Read the model definition and answer for the solid it produces. Units are mm, in the model's axes. A direction names the side the tool comes from. Round coordinates to 2 decimals unless told otherwise and drop trailing zeros. Write each loop counter-clockwise with the first axis right and the second up, starting at its lowest first coordinate (ties: lowest second). Pieces come first, ordered by that corner, then holes. Notation, with made-up numbers: (52.5, 2.25) -> (63.5, 2.25) arc R25 ccw to (63.5, 27.25) -> close; hole circle Ø3 at (85, 34). An arc over 180 degrees is marked (long way). Return JSON: item names as keys, results as strings.
Autodesk Inventor part; units mm, degrees
ref_plane "YZ Plane" through (0, 0, 0) normal (1, 0, 0) x (0, 1, 0)
ref_plane "XZ Plane" through (0, 0, 0) normal (0, 1, 0) x (-1, 0, 0)
ref_plane "XY Plane" through (0, 0, 0) normal (0, 0, 1) x (1, 0, 0)
sketch "스케치1" plane through (0, 0, 0) normal (0, 1, 0) x (-1, 0, 0)
  line L0 (17.6385, -30.5508) -> (-17.6385, -30.5508)
  line L1 (-17.6385, -30.5508) -> (-35.277, 0)
  line L2 (-35.277, 0) -> (-17.6385, 30.5508)
  line L3 (-17.6385, 30.5508) -> (17.6385, 30.5508)
  line L4 (17.6385, 30.5508) -> (35.277, 0)
  line L5 (35.277, 0) -> (17.6385, -30.5508)
  line L6 (19.486, -33.7508) -> (-19.486, -33.7508)
  line L7 (-19.486, -33.7508) -> (-38.972, 0)
  line L8 (-38.972, 0) -> (-19.486, 33.7508)
  line L9 (-19.486, 33.7508) -> (19.486, 33.7508)
  line L10 (19.486, 33.7508) -> (38.972, 0)
  line L11 (38.972, 0) -> (19.486, -33.7508)
  point P0 (0, 0)
  point P1 (0, 0)
  point P2 (0, 0)
  dimension "d0" = 70.554
  dimension "d1" = 3.2
extrude "돌출1" add sketch "스케치1" along normal blind 3.7 contours L0 L1 L2 L3 L4 L5 | L6 L7 L8 L9 L10 L11
sketch "스케치2" plane through (0, 3.7, 0) normal (0, 1, 0) x (1, 0, 0)
  line L0 (-18.5623, 32.1508) -> (18.5623, 32.1508)
  line L1 (18.5623, 32.1508) -> (37.1245, 0)
  line L2 (37.1245, 0) -> (18.5623, -32.1508)
  line L3 (18.5623, -32.1508) -> (-18.5623, -32.1508)
  line L4 (-18.5623, -32.1508) -> (-37.1245, 0)
  line L5 (-37.1245, 0) -> (-18.5623, 32.1508)
  line L6 (-19.486, 33.7508) -> (-38.972, 0)
  point P0 (0, 0)
  point P1 (0, 0)
  dimension "d4" = 1.6
extrude "돌출2" cut sketch "스케치2" against normal blind 1.2
sketch "스케치3" plane through (0, 2.5, 0) normal (0, 1, 0) x (1, 0, 0)
  line L0 (17.4076, -30.1508) -> (-17.4076, -30.1508)
  line L1 (-17.4076, -30.1508) -> (-34.8151, 0)
  line L2 (-34.8151, 0) -> (-17.4076, 30.1508)
  line L3 (-17.4076, 30.1508) -> (17.4076, 30.1508)
  line L4 (17.4076, 30.1508) -> (34.8151, 0)
  line L5 (34.8151, 0) -> (17.4076, -30.1508)
  line L6 (-18.5623, 32.1508) -> (18.5623, 32.1508)
  point P0 (0, 0)
  point P1 (0, 0)
  dimension "d7" = 2
extrude "돌출3" add sketch "스케치3" along normal blind 0.6
fillet "모깎기1" radius 1.2 12 edges at (0, 3.7, -33.7508) (0, 0, -33.7508) (-29.229, 3.7, -16.8754) (-29.229, 0, -16.8754) (-29.229, 3.7, 16.8754) (-29.229, 0, 16.8754) (0, 0, 33.7508) (0, 3.7, 33.7508) (29.229, 0, 16.8754) (29.229, 3.7, 16.8754) (29.229, 3.7, -16.8754) (29.229, 0, -16.8754)
sketch "스케치10" plane through (0, 0, 0) normal (0, -1, 0) x (1, 0, 0)
  line L0 (-12.5, 15.3) -> (12.5, 15.3)
  line L1 (12.5, 15.3) -> (12.5, 10.3)
  line L2 (12.5, 10.3) -> (-12.5, 10.3)
  line L3 (-12.5, 10.3) -> (-12.5, 15.3)
  line L4 (-12.5, 15.3) -> (12.5, 10.3) construction
  line L5 (12.5, 15.3) -> (-12.5, 10.3) construction
  line L6 (0, 0) -> (7.4968, 0)
  line L7 (-12.5, -15.3) -> (12.5, -15.3)
  line L8 (12.5, -15.3) -> (12.5, -10.3)
  line L9 (12.5, -10.3) -> (-12.5, -10.3)
  line L10 (-12.5, -10.3) -> (-12.5, -15.3)
  line L11 (-12.5, -15.3) -> (12.5, -10.3) construction
  line L12 (12.5, -15.3) -> (-12.5, -10.3) construction
  point P0 (0, 12.8)
  point P1 (0, -12.8)
  dimension "d51" = 25
  dimension "d52" = 5
  dimension "d53" = 10.3
extrude "돌출7" add sketch "스케치10" along normal blind 15
sketch "스케치11" plane through (12.5, 0, -15.3) normal (0, 0, -1) x (-1, 0, 0)
  circle A0 centre (7.5, -7.5) radius 1.25
  line L0 (-6.2932, 0) -> (31.2932, 0)
  line L1 (12.5, 0) -> (12.5, -3.2028)
  circle A1 centre (17.5, -7.5) radius 1.25
  point P0 (12.5, 0)
  dimension "d56" = 2.5
  dimension "d57" = 7.5
  dimension "d58" = 5
extrude "돌출8" cut sketch "스케치11" against normal up to surface (30.6 mm away)
properties part number "OV-PAM_n_6_bottom"
Item 1: Flat-ended cylindrical pins translate along their axes: pin 1 (0.5 mm diameter, centred on x = 0, y = 3, fed in from -Z); pin 2 (1 mm diameter, centred on x = -14, z = 5, fed in from -Y); pin 3 (2 mm diameter, centred on x = -4.5, y = -9.5, fed in from +Z); pin 4 (2 mm diameter, centred on x = -5, y = -7.5, fed in from +Z). Find the tip coordinate at first contact, or state that the pin passes through.
Worked answers:
{"pin 1": "stops at z = -33.72", "pin 2": "stops at y = 0", "pin 3": "stops at z = 15.3", "pin 4": "passes through"}
Item 2: Straight lines are drawn through the part: L1, parallel to Y at x = -5, z = 14; L2, parallel to Z at x = 12, y = -4.5; L3, parallel to Y at x = -10, z = 12. For each, find the intervals that lie inside material, in ascending order. Write a range as [from, to].
Worked answers:
{"L1": "y = [-15, -8.75], [-6.25, 3.1]", "L2": "z = [-15.3, -10.3], [10.3, 15.3]", "L3": "y = [-15, 3.1]"}
Item 3: For a pull along Z with two mould halves and no side action, classify faces 1 (the flat face through (27.713, 3.108, -16.3)), 2 (the cylindrical face through (-4.73, -8.72, 12.76)), 3 (the flat face through (-27.973, 3.108, -15.85)), 4 (the flat face through (0, -7, -15.3)) as released by +Z, released by -Z, zero draft, split by the parting line, or undercut.
Worked answers:
{"face 1": "undercut", "face 2": "zero draft", "face 3": "undercut", "face 4": "released by -Z"}
Item 4: A tool of negligible diameter and unlimited length cuts with its end or side. For faces 5 (the flat face through (0, -7, 15.3)), 6 (the flat face through (12.5, -7, 13)), 7 (the flat face through (-12.5, -7, 13)), from which of +Z, -Z, +X, -X, +Y, -Y can it reach the whole face along a straight path? Write none if from no direction.
Worked answers:
{"face 5": "+Z, +X, -X, -Y", "face 6": "+Z, -Z, +X, -Y", "face 7": "+Z, -Z, -X, -Y"}
Item 5: Section B-B (y = -7.5) is taken. Give the vertices of the cut face in (x, z), then the cut area to 3 significant figures.
Worked answers:
{"outline": "(-12.5, -15.3) -> (-6.25, -15.3) -> (-6.25, -10.3) -> (-12.5, -10.3) -> close; (-12.5, 10.3) -> (-6.25, 10.3) -> (-6.25, 15.3) -> (-12.5, 15.3) -> close; (-3.75, -15.3) -> (3.75, -15.3) -> (3.75, -10.3) -> (-3.75, -10.3) -> close; (-3.75, 10.3) -> (3.75, 10.3) -> (3.75, 15.3) -> (-3.75, 15.3) -> close; (6.25, -15.3) -> (12.5, -15.3) -> (12.5, -10.3) -> (6.25, -10.3) -> close; (6.25, 10.3) -> (12.5, 10.3) -> (12.5, 15.3) -> (6.25, 15.3) -> close", "area": "200 mm2"}
Item 6: Section A-A (x = 5) is taken. State how many separate pieces and enclosed holes the cut face has, then the cut area to 3 significant figures.
Worked answers:
{"separate pieces": "3", "enclosed holes": "0", "area": "333 mm2"}
Item 7: Section C-C (y = -11.25) is taken. Give the vertices of the cut face in (x, z), then the cut area to 3 significant figures.
Worked answers:
{"outline": "(-12.5, -15.3) -> (12.5, -15.3) -> (12.5, -10.3) -> (-12.5, -10.3) -> close; (-12.5, 10.3) -> (12.5, 10.3) -> (12.5, 15.3) -> (-12.5, 15.3) -> close", "area": "250 mm2"}
